from build123d import *

# Parameters (mm, degrees)
SKETCH2_W               = 63.52
SKETCH2_H               = 30.59
BOSS_EXTRUDE1_DEPTH     = 7
SKETCH3_W               = 3
SKETCH3_H               = 30.59
BOSS_EXTRUDE2_DEPTH     = 40
FILLET2_R               = 3
SKETCH4_R               = 1.25
CUT_EXTRUDE2_DEPTH      = 70
CUT_EXTRUDE4_DEPTH      = 20
CUT_EXTRUDE4_DEPTH_BACK = 6
SKETCH7_R               = 1.25


with BuildPart() as part:
    # Sketch2 → Boss-Extrude1 (new body)
    with BuildSketch(Plane(origin=(0, 0, 0), x_dir=(1, 0, 0), z_dir=(0, 1, 0))):
        with Locations((-20.26308022, 14.924105874)):
            Rectangle(SKETCH2_W, SKETCH2_H)
    extrude(amount=BOSS_EXTRUDE1_DEPTH)

    # Sketch3 → Boss-Extrude2 (add)
    with BuildSketch(Plane(origin=(0, 7, 0), x_dir=(1, 0, 0), z_dir=(0, 1, 0))):
        with Locations((-50.52308022, 14.924105874)):
            Rectangle(SKETCH3_W, SKETCH3_H)
        with Locations((9.99691978, 14.924105874)):
            Rectangle(SKETCH3_W, SKETCH3_H)
    extrude(amount=BOSS_EXTRUDE2_DEPTH)

    # Fillet2
    fillet2_edges = [part.edges().sort_by_distance(p)[0] for p in [
        (11.49691978, 0, -14.924105874),
        (-52.02308022, 0, -14.924105874),
    ]]
    fillet(fillet2_edges, radius=FILLET2_R)

    # Sketch4 → Cut-Extrude2 (cut)
    with BuildSketch(Plane.ZY.offset(52.02308022)):
        with BuildLine():
            Line((-30.219105874, 47), (-30.219105874, 3))
            Line((-30.219105874, 3), (-25.063958288, 35.226112217))
            ThreePointArc((-25.063958288, 35.226112217), (-14.924105874, 43.987089872), (-4.784253461, 35.226112217))
            Line((-4.784253461, 35.226112217), (0.370894126, 3))
            Line((0.370894126, 3), (0.370894126, 47))
            Line((0.370894126, 47), (-30.219105874, 47))
        make_face()
        with Locations((-7.424105874, 33.73872813)):
            Circle(SKETCH4_R)
        with Locations((-7.424105874, 30.23872813)):
            Circle(SKETCH4_R)
        with Locations((-7.424105874, 36.73872813)):
            Circle(SKETCH4_R)
        with Locations((-14.924105874, 26.23872813)):
            Circle(SKETCH4_R)
        with Locations((-11.424105874, 26.23872813)):
            Circle(SKETCH4_R)
        with Locations((-18.424105874, 26.23872813)):
            Circle(SKETCH4_R)
        with Locations((-22.424105874, 33.73872813)):
            Circle(SKETCH4_R)
        with Locations((-22.424105874, 37.23872813)):
            Circle(SKETCH4_R)
        with Locations((-22.424105874, 30.23872813)):
            Circle(SKETCH4_R)
        with Locations((-11.424105874, 41.23872813)):
            Circle(SKETCH4_R)
        with Locations((-18.424105874, 41.23872813)):
            Circle(SKETCH4_R)
        with Locations((-14.924105874, 41.23872813)):
            Circle(SKETCH4_R)
    extrude(amount=-CUT_EXTRUDE2_DEPTH, mode=Mode.SUBTRACT)

    # Sketch7 → Cut-Extrude4 (cut, two sides: drawn at the far end of the back side and taken through both)
    with BuildSketch(Plane(origin=(0, 0, 0), x_dir=(1, 0, 0), z_dir=(0, 1, 0)).offset(-CUT_EXTRUDE4_DEPTH_BACK)):
        with Locations(Location((-20.263080223, 21.924105874, 0), (0, 0, 270))):
            Circle(SKETCH7_R)
        with Locations(Location((-20.263080223, 6.924105874, 0), (0, 0, 270))):
            Circle(SKETCH7_R)
        with Locations(Location((-12.763080223, 14.424105874, 0), (0, 0, 270))):
            Circle(SKETCH7_R)
        with Locations(Location((-27.763080223, 14.424105874, 0), (0, 0, 270))):
            Circle(SKETCH7_R)
        with Locations(Location((-12.763080223, 17.924105874, 0), (0, 0, 270))):
            Circle(SKETCH7_R)
        with Locations(Location((-12.763080223, 10.924105874, 0), (0, 0, 270))):
            Circle(SKETCH7_R)
        with Locations(Location((-16.763080223, 6.924105874, 0), (0, 0, 270))):
            Circle(SKETCH7_R)
        with Locations(Location((-23.763080223, 6.924105874, 0), (0, 0, 270))):
            Circle(SKETCH7_R)
        with Locations(Location((-16.763080223, 21.924105874, 0), (0, 0, 270))):
            Circle(SKETCH7_R)
        with Locations(Location((-23.763080223, 21.924105874, 0), (0, 0, 270))):
            Circle(SKETCH7_R)
        with Locations(Location((-27.763080223, 17.924105874, 0), (0, 0, 270))):
            Circle(SKETCH7_R)
        with Locations(Location((-27.763080223, 10.924105874, 0), (0, 0, 270))):
            Circle(SKETCH7_R)
    extrude(amount=CUT_EXTRUDE4_DEPTH + CUT_EXTRUDE4_DEPTH_BACK, mode=Mode.SUBTRACT)


solid = part.part
The listing builds one solid part. Answer for the finished solid, in the listing's coordinates (mm). Give positions to 0.01 mm unless a question says otherwise; leave off trailing zeros. Loops run counter-clockwise (first coordinate to the right, second up) from the corner with the lowest first, then second, coordinate; pieces in that order, holes last. Notation, with made-up numbers: M 28,77 L 66,77 A19 cw 66,95 Z; hole C -4,59.5 d7. An arc over 180 degrees is marked long. Answer as CSV lines item,"result".
Item 1: The part is cut by section A-A (y = 9). Give the vertices of the cut face in (x, z), and give its area (3 significant figures).
Values follow:
outline,"M -52.02,-29.26 L -49.02,-29.26 L -49.02,-0.59 L -52.02,-0.59 Z; M 8.5,-29.26 L 11.5,-29.26 L 11.5,-0.59 L 8.5,-0.59 Z"
area,"172 mm^2"
Item 2: The mould has two halves that part along X. Classify faces 1 (the cylindrical face through (9.976, 43.985, -15.129)), 2 (the cylindrical face through (-21.483, 3.451, -7.195)), 3 (the cylindrical face through (-17.983, 3.451, -22.195)), 4 (the cylindrical face through (-51.168, 0.902, -15.138)): released by +X, released by -X, zero draft, split by the parting line, or undercut.
Values follow:
face 1,"zero draft"
face 2,"undercut"
face 3,"undercut"
face 4,"released by -X"
Item 3: The part is cut by section C-C (x = 3.5). Give the vertices of the cut face in (y, z).
Values follow:
outline,"M 0,-30.22 L 3,-30.22 L 7,-29.58 L 7,-0.27 L 3,0.37 L 0,0.37 Z"
Item 4: The part is cut by section B-B (z = -15). Give the number of separate pieces and of enclosed holes in the cut face, and give its area (3 significant figures).
Values follow:
separate pieces,"7"
enclosed holes,"0"
area,"602 mm^2"
Item 5: Straight lines are drawn through the part: line 1 along X through (y, z) = (12.5, -10.5); line 2 along X through (y, z) = (4, -22); line 3 along X through (y, z) = (6, -6.5). For each, find the intervals that lie inside material, in ascending order. Write a range as [from, to].
Values follow:
line 1,"x = [-52.02, -49.02], [8.5, 11.5]"
line 2,"x = [-52.02, -25.01], [-22.52, -21.51], [-19.02, -18.01], [-15.52, 11.5]"
line 3,"x = [-52.02, -24.94], [-22.59, -21.44], [-19.09, -17.94], [-15.59, 11.5]"
Item 6: The part is cut by section D-D (z = -1.5). Give the vertices of the cut face in (x, y).
Values follow:
outline,"M -52.02,3 A3 ccw -49.02,0 L 8.5,0 A3 ccw 11.5,3 L 11.5,14.7 L 8.5,14.7 L 8.5,7 L -49.02,7 L -49.02,14.7 L -52.02,14.7 Z"
Item 7: Given pin 1 Ø1.5 at (y, z) = (26.24, -18.42) entering from +X; pin 2 Ø3 at (x, z) = (-14, -20.5) entering from +Y, each flat-ended and moving along its own axis, determine where each tip first touches the part or whether it passes through.
Values follow:
pin 1,"passes through"
pin 2,"stops at y = 7"
